For this review, use the dimensioned drawing (mm, ordinates from the lowest corner) and the shaded views. Give positions to 0.01 mm unless a question says otherwise; leave off trailing zeros. Loops run counter-clockwise (first coordinate to the right, second up) from the corner with the lowest first, then second, coordinate; pieces in that order, holes last. Notation, with made-up numbers: M 88,-5 L 105,-5 A9 ccw 105,3 Z; hole C 24.5,26 d2. An arc over 180 degrees is marked long. Use a Markdown table: item, result. Add a question column.
(1) Add section A-A, the plane z = 15.5. Give the boundary of the cut face in (x, y), then the cut area to 3 significant figures.
(2) Add section D-D, the plane z = 124. Give the boundary of the cut face in (x, y), then the cut area to 3 significant figures.
(3) For probe 1 along Y at (x, z) = (3.25, 135.5); probe 2 along Y at (x, z) = (4, 57); probe 3 along Y at (x, z) = (1.75, 65), list the stretches that pass through material, from the lowest coordinate up.
(4) Insertion check: pin 1 Ø3 at (x, z) = (5.5, 125) entering from +Y; pin 2 Ø3 at (x, z) = (2.5, 154.5) entering from +Y. Each pin has a flat end and moves straight along its axis. Give the tip position at first contact, or say it passes through.
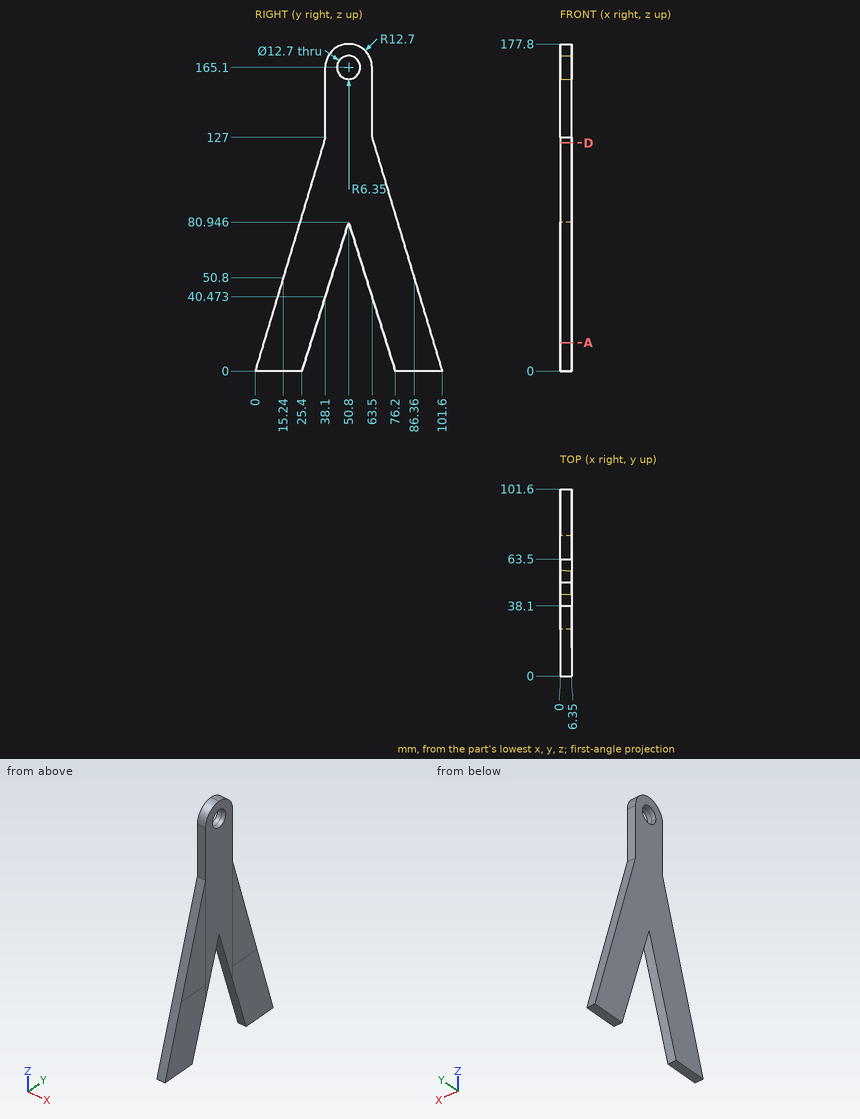
Established:
| question | item | result |
|---|---|---|
| 1 | outline | M 0,4.65 L 6.35,4.65 L 6.35,30.26 L 0,30.26 Z; M 0,71.34 L 6.35,71.34 L 6.35,96.95 L 0,96.95 Z |
| 1 | area | 325 mm^2 |
| 2 | outline | M 0,37.2 L 6.35,37.2 L 6.35,64.4 L 0,64.4 Z |
| 2 | area | 173 mm^2 |
| 3 | probe 1 | 38.1 to 63.5 |
| 3 | probe 2 | 17.1 to 43.29, 58.31 to 84.5 |
| 3 | probe 3 | 19.5 to 45.8, 55.8 to 82.1 |
| 4 | pin 1 | y = 64.55 |
| 4 | pin 2 | y = 63.5 |
